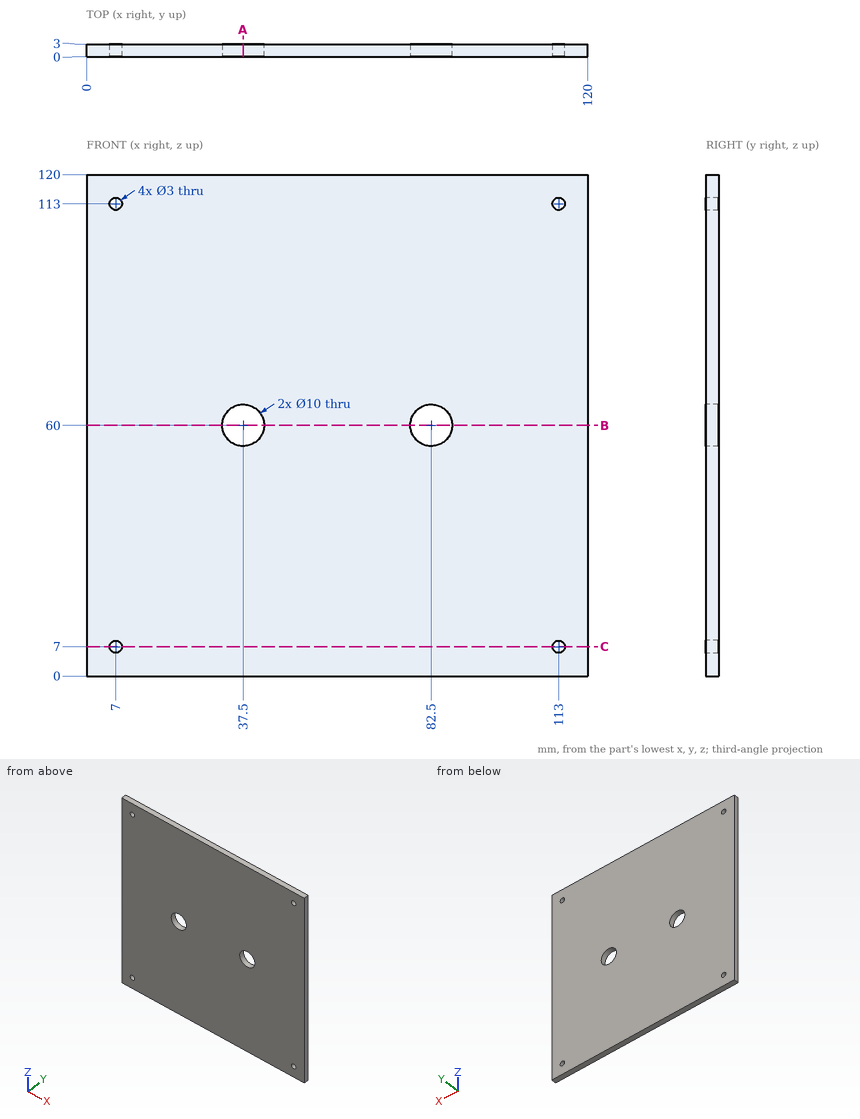
The drawing under review shows one solid part. Ordinate dimensions are in mm from its lowest x, y, z. Coordinates: 2 decimals unless noted, no trailing zeros. Write each loop counter-clockwise with the first axis right and the second up, starting at its lowest first coordinate (ties: lowest second). Pieces come first, ordered by that corner, then holes. Notation, with made-up numbers: M -20.75,10.25 L 9.25,10.25 A15 ccw 9.25,21.25 Z; hole C -12.75,71.5 d10. An arc over 180 degrees is marked long. Put each result on its own line as item: value.
1) Add section C-C on z = 7. Give the boundary of the cut face in (x, y), then the cut area to 3 significant figures.
Computed:
outline: M 0,0 L 5.5,0 L 5.5,3 L 0,3 Z; M 8.5,0 L 111.5,0 L 111.5,3 L 8.5,3 Z; M 114.5,0 L 120,0 L 120,3 L 114.5,3 Z
area: 342 mm2
2) Add section A-A on x = 37.5. Give the boundary of the cut face in (y, z).
Computed:
outline: M 0,0 L 3,0 L 3,55 L 0,55 Z; M 0,65 L 3,65 L 3,120 L 0,120 Z
3) Clearance check with a flat-ended pin moving along its axis: pin 1 Ø13 at (x, z) = (37.5, 60) entering from -Y. State where the tip first meets the part, or that it passes through.
Computed:
pin 1: stops at y = 0
4) Wall thickness on probe 1 along X at (y, z) = (0.7, 60); probe 2 along Z at (x, y) = (113, 0.7); probe 3 along X at (y, z) = (1.05, 63): over which ranges is each line inside the solid? List them lowest first. Write a range as [from, to].
Computed:
probe 1: x = [0, 32.5], [42.5, 77.5], [87.5, 120]
probe 2: z = [0, 5.5], [8.5, 111.5], [114.5, 120]
probe 3: x = [0, 33.5], [41.5, 78.5], [86.5, 120]
5) Add section B-B on z = 60. Give the boundary of the cut face in (x, y).
Computed:
outline: M 0,0 L 32.5,0 L 32.5,3 L 0,3 Z; M 42.5,0 L 77.5,0 L 77.5,3 L 42.5,3 Z; M 87.5,0 L 120,0 L 120,3 L 87.5,3 Z
